Input: dimensioned drawing with shaded views. Units: mm. Origin: part minimum x, y, z. A direction names the side the tool comes from. Round coordinates to 2 decimals unless told otherwise and drop trailing zeros. Loops run counter-clockwise (first coordinate to the right, second up) from the corner with the lowest first, then second, coordinate; pieces in that order, holes last. Notation, with made-up numbers: M 8.5,18.5 L 22.5,18.5 A20 ccw 22.5,57.5 Z; hole C 41,57.5 d6. An arc over 180 degrees is marked long. Answer as a JSON object with one key per item and string values.
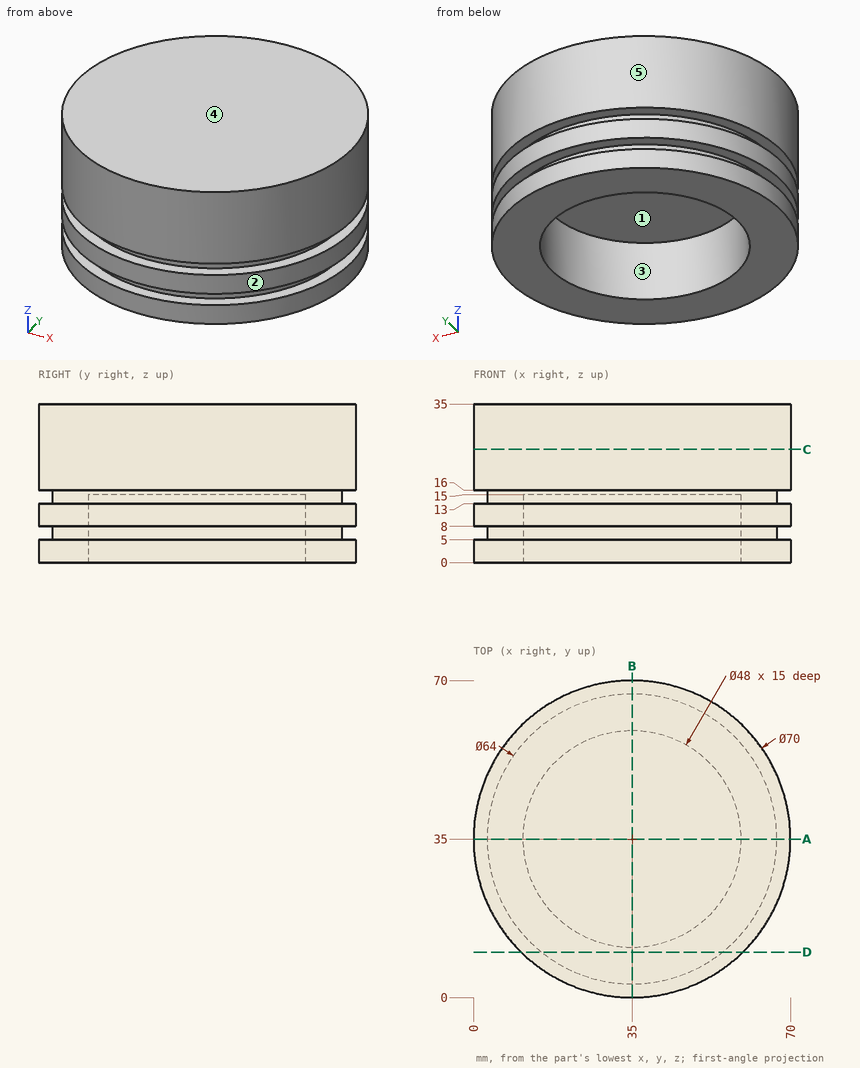
Item 1: Section D-D on y = 10. Return the cut outline in (x, z), then the cut area to 3 significant figures.
Answer sheet:
{"outline": "M 10.51,0 L 59.49,0 L 59.49,5 L 54.97,5 L 54.97,8 L 59.49,8 L 59.49,13 L 54.97,13 L 54.97,16 L 59.49,16 L 59.49,35 L 10.51,35 L 10.51,16 L 15.03,16 L 15.03,13 L 10.51,13 L 10.51,8 L 15.03,8 L 15.03,5 L 10.51,5 Z", "area": "1,660 mm²"}
Item 2: Section A-A on y = 35. Return the cut outline in (x, z), then the cut area to 3 significant figures.
Answer sheet:
{"outline": "M 0,0 L 11,0 L 11,15 L 59,15 L 59,0 L 70,0 L 70,5 L 67,5 L 67,8 L 70,8 L 70,13 L 67,13 L 67,16 L 70,16 L 70,35 L 0,35 L 0,16 L 3,16 L 3,13 L 0,13 L 0,8 L 3,8 L 3,5 L 0,5 Z", "area": "1,690 mm²"}
Item 3: Access query for the marked faces 1 and 2. Directions: +Z, -Z, +X, -X, +Y, -Y. A direction counts if a zero-diameter tool reaches every point of the face in a straight line with its end or side. Return the directions, or none.
Answer sheet:
{"face 1": "-Z", "face 2": "+Z, -Z"}
Item 4: Contact query for flat-ended pins moving along their axis: pin 1 Ø2 at (x, z) = (32.5, 31) entering from +Y; pin 2 Ø4 at (y, z) = (15.5, 10) entering from +X; pin 3 Ø1.5 at (y, z) = (54, 23) entering from +X. Output: stop coordinate, or through.
Answer sheet:
{"pin 1": "stops at y = 69.97", "pin 2": "stops at x = 65.31", "pin 3": "stops at x = 64.87"}
Item 5: Section C-C on z = 25. Return the cut outline in (x, y), then the cut area to 3 significant figures.
Answer sheet:
{"outline": "C 35,35 d70", "area": "3,850 mm²"}
Item 6: Pull-direction query (Y, two-part tool) for the marked faces 3, 4 and 5; classes: pulls with the +Y half, pulls with the -Y half, needs draft (parallel to the pull), parting line crosses it, or undercut.
Answer sheet:
{"face 3": "undercut", "face 4": "needs draft", "face 5": "parting line crosses it"}
Item 7: Line query: probe 1 along Z at (x, y) = (8, 54); probe 2 along X at (y, z) = (35, 8.5); probe 3 along X at (y, z) = (35, 6). Output: solid intervals per line, ascending. Write a range as from..to.
Answer sheet:
{"probe 1": "z = 0..5, 8..13, 16..35", "probe 2": "x = 0..11, 59..70", "probe 3": "x = 3..11, 59..67"}
